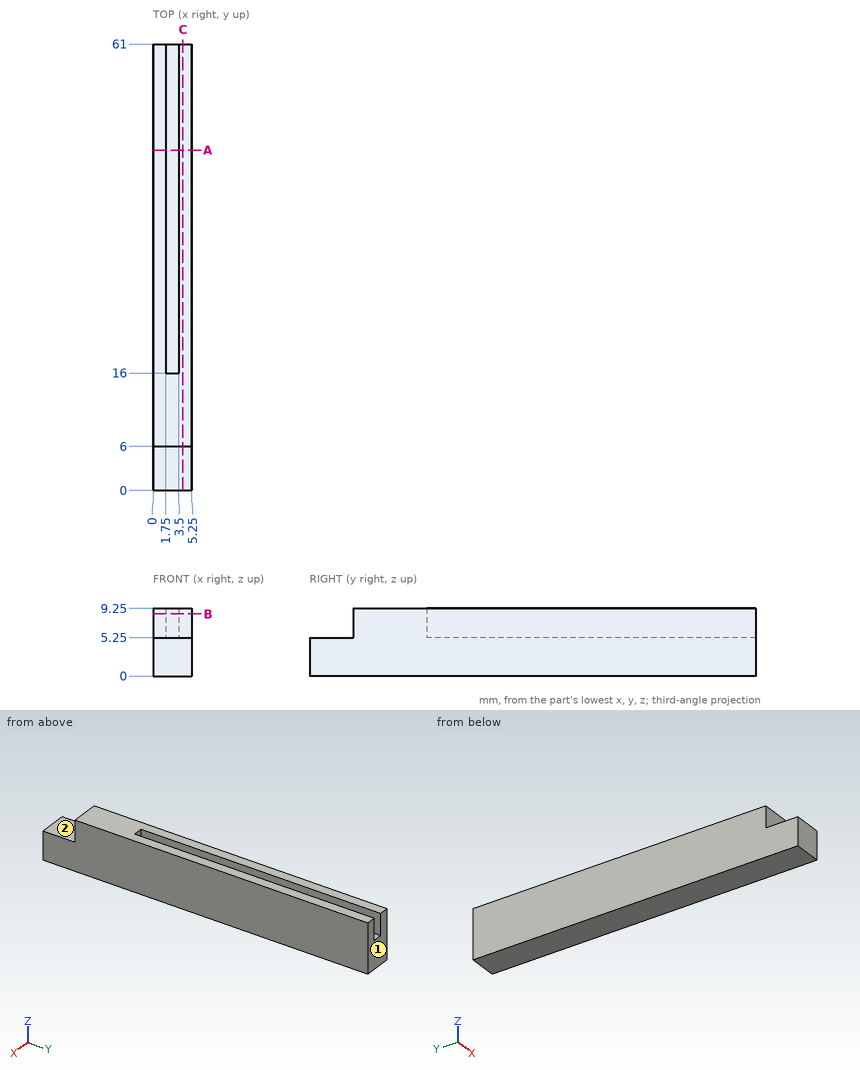
Input: dimensioned drawing with shaded views. Units: mm. Origin: part minimum x, y, z. A direction names the side the tool comes from. Coordinates: 2 decimals unless noted, no trailing zeros. Order: outer loops, then holes, each group sorted by start corner. A loop starts at its lowest first (then second) coordinate and runs counter-clockwise, first axis right, second up. Notation, with made-up numbers: (-7, 60.5) -> (52, 60.5) arc R22 ccw to (52, 77.5) -> close; hole circle Ø4 at (3, -26). An arc over 180 degrees is marked (long way). Use CSV: the item, a comma, the result in double quotes.
1) Access query for the marked faces 1 and 2. Directions: +Z, -Z, +X, -X, +Y, -Y. A direction counts if a zero-diameter tool reaches every point of the face in a straight line with its end or side. Return the directions, or none.
Findings:
face 1,"+Z, -Z, +X, -X, +Y"
face 2,"+Z, +X, -X, -Y"
2) Section B-B on z = 8.5. Output: boundary loops of the cut face in (x, y), then the cut area to 3 significant figures.
Findings:
outline,"(0, 6) -> (5.25, 6) -> (5.25, 61) -> (3.5, 61) -> (3.5, 16) -> (1.75, 16) -> (1.75, 61) -> (0, 61) -> close"
area,"210 mm^2"
3) Section C-C on x = 4.05. Output: boundary loops of the cut face in (y, z).
Findings:
outline,"(0, 0) -> (61, 0) -> (61, 9.25) -> (6, 9.25) -> (6, 5.25) -> (0, 5.25) -> close"
4) Pin query (flat end, axial travel): pin 1 Ø2.5 at (x, y) = (3, 2.5) entering from +Z; pin 2 Ø1.4 at (x, z) = (2.5, 8) entering from +Y. Return the tip coordinate at first contact, or that it passes through.
Findings:
pin 1,"stops at z = 5.25"
pin 2,"stops at y = 16"
5) Section A-A on y = 46.5. Output: boundary loops of the cut face in (x, z), then the cut area to 3 significant figures.
Findings:
outline,"(0, 0) -> (5.25, 0) -> (5.25, 9.25) -> (3.5, 9.25) -> (3.5, 5.25) -> (1.75, 5.25) -> (1.75, 9.25) -> (0, 9.25) -> close"
area,"41.6 mm^2"
6) Line query: line 1 (X direction, y = 43, z = 7.25); line 2 (Y direction, x = 0.3, z = 5.75); line 3 (Y direction, x = 2.8, z = 5.5). Output: solid intervals per line, ascending.
Findings:
line 1,"x = 0 to 1.75, 3.5 to 5.25"
line 2,"y = 6 to 61"
line 3,"y = 6 to 16"
